Read the model definition and answer for the solid it produces. Units are mm, in the model's axes. Give positions to 0.01 mm unless a question says otherwise; leave off trailing zeros. Write each loop counter-clockwise with the first axis right and the second up, starting at its lowest first coordinate (ties: lowest second). Pieces come first, ordered by that corner, then holes. Notation, with made-up numbers: (50, -2) -> (76, -2) arc R17 cw to (76, 10) -> close; hole circle Ø4 at (78, 24.25). An arc over 180 degrees is marked (long way). Use a Markdown table: item, result.
from build123d import *
from build123d import SkipClean  # not in build123d's __all__


# Not quite as in the source:
# - ends of sketch curves that miss each other by under 0.0002 mm in the source are joined


with BuildPart() as f1:
    # F0 (on Front) → F1 (revolve)
    with BuildSketch(Plane.XZ):
        with BuildLine():
            ThreePointArc((150, 0), (152.3425507406, 15.1250629778), (159.1507012033, 28.8328768565))
            Line((159.1507012033, 28.8328768565), (199.542465, 86.058356))
            ThreePointArc((199.542465, 86.058356), (199.7196970287, 88.6501935058), (197.5, 90))
            Line((197.5, 90), (0, 90))
            Line((0, 90), (0, 0))
            Line((0, 0), (150, 0))
        make_face()
    revolve(axis=Axis((0, 0, 45), (0, 0, 1)))

    # F2: F1 across face


with BuildPart() as f1_1:
    add(f1.part, clean=False)
    with SkipClean():  # cleaning this boolean's faces spoils the solid; the shape is the same uncleaned
        add(f1.part.mirror(Plane(origin=(0, 0, 0), x_dir=(1, 0, 0), z_dir=(0, 0, -1))), clean=False)


solid = f1_1.part
Item 1: A cutting plane is placed at A-A (z = -16). Give the vertices of the cut face in (x, y).
Return value:
| item | result |
|---|---|
| outline | circle Ø305.26 at (0, 0) |
Item 2: For a pull along Z with two mould halves and no side action, classify faces 1 (the face through (-3, 3, 90)), 2 (the face through (-35.05, -157.83, -32.41)), 3 (the face through (-3, 3, -90)) as +Z half, -Z half, draft (parallel to the pull), parting line (faces both ways), or undercut.
Return value:
| item | result |
|---|---|
| face 1 | +Z half |
| face 2 | undercut |
| face 3 | -Z half |
Item 3: Straight lines are drawn through the part: line 1 along Z through (x, y) = (-147, 65); line 2 along Z through (x, y) = (-175, 56); line 3 along X through (y, z) = (4, 30). For each, find the intervals that lie inside material, in ascending order. Write a range as [from, to].
Return value:
| item | result |
|---|---|
| line 1 | [-90, -31.07], [31.07, 90] |
| line 2 | [-90, -63.67], [63.67, 90] |
| line 3 | [-159.92, 159.92] |
Item 4: Each of these flat-tipped pins is pushed along its axis until it touches: P1, Ø6, axis at y = -20.5, z = -39, coming from the +X side; P2, Ø1, axis at x = -34.5, z = 6.5, coming from the -Y side; P3, Ø8, axis at x = -131, z = -63, coming from the +Y side. Where does it stop, or does it pass through?
Return value:
| item | result |
|---|---|
| P1 | x = 167.22 |
| P2 | y = -146.55 |
| P3 | y = 133.77 |
